Can you work these out from the model? Positions are in its coordinate system, mm. Give positions to 0.01 mm unless a question says otherwise; leave off trailing zeros. Loops run counter-clockwise (first coordinate to the right, second up) from the corner with the lowest first, then second, coordinate; pieces in that order, holes last. Notation, with made-up numbers: (66.5, 48) -> (90.5, 48) arc R10 ccw to (90.5, 53) -> close; hole circle Ø2 at (19.5, -3.5). An arc over 180 degrees is marked (long way). Return JSON: item names as keys, results as strings. Group by question number.
Q1. Suppose I cut it at A-A, the plane y = 0. Please give me the cut outline in (x, z), and give its area (3 significant figures).
Q2. Suppose I cut it at B-B, the plane x = 0. Please give me the cut outline in (y, z), and give its area (3 significant figures).
Q3. I need wall thicknesses on line 1 along Y through (x, z) = (0, 16); line 2 along X through (y, z) = (-7, 28.75); line 3 along Y through (x, z) = (-132.5, 5.5). Which ranges of each line are inside material? Lowest first, please. Write a range as [from, to].
```python
from build123d import *

# Parameters (mm, degrees)
ESBO_O1_W                = 550
ESBO_O1_H                = 400
ESBO_O1_R                = 12
RESSALTO_EXTRUS_O1_DEPTH = 30


with BuildPart() as part:
    # Esboço1 → Ressalto-extrusão1 (new body)
    with BuildSketch(Plane.XY):
        Rectangle(ESBO_O1_W, ESBO_O1_H)
        with Locations((-129.722465626, 52.650564213)):
            Circle(ESBO_O1_R, mode=Mode.SUBTRACT)
        Circle(ESBO_O1_R, mode=Mode.SUBTRACT)
        with Locations((134.18182058, 39.940443486)):
            Circle(ESBO_O1_R, mode=Mode.SUBTRACT)
    extrude(amount=RESSALTO_EXTRUS_O1_DEPTH)


solid = part.part
```
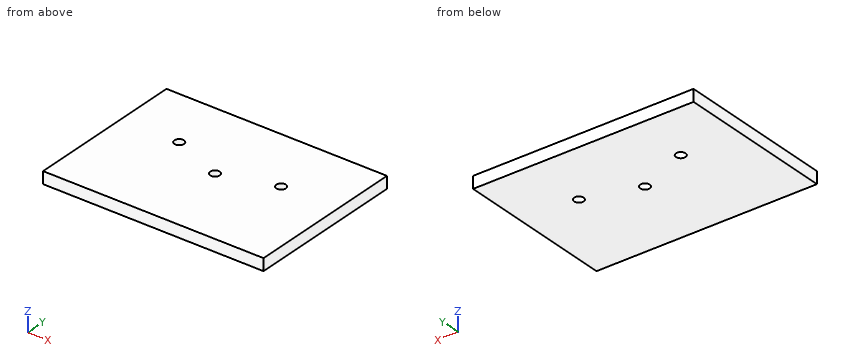
Ans:
{
 "1": {"outline": "(-275, 0) -> (-12, 0) -> (-12, 30) -> (-275, 30) -> close; (12, 0) -> (275, 0) -> (275, 30) -> (12, 30) -> close", "area": "15,800 mm^2"},
 "2": {"outline": "(-200, 0) -> (-12, 0) -> (-12, 30) -> (-200, 30) -> close; (12, 0) -> (200, 0) -> (200, 30) -> (12, 30) -> close", "area": "11,300 mm^2"},
 "3": {"line 1": "y = [-200, -12], [12, 200]", "line 2": "x = [-275, -9.75], [9.75, 275]", "line 3": "y = [-200, 40.98], [64.32, 200]"}
}
